The model under review builds one solid part; all positions refer to its coordinate system, in mm. A direction names the side the tool comes from. Coordinates: 2 decimals unless noted, no trailing zeros. Order: outer loops, then holes, each group sorted by start corner. A loop starts at its lowest first (then second) coordinate and runs counter-clockwise, first axis right, second up.
```python
from build123d import *

# Parameters (mm, degrees)
SKETCH_1_W          = 10
SKETCH_1_H          = 10
SKETCH_1_W_2        = 8
SKETCH_1_H_2        = 8
EXTRUDE_1_DEPTH     = 52.5
SKETCH_2_R          = 1.6
CUT_EXTRUDE_1_DEPTH = 54.677276384
SKETCH_3_R          = 1.6
CUT_EXTRUDE_2_DEPTH = 54.677276384
SKETCH_4_R          = 1.6
CUT_EXTRUDE_3_DEPTH = 54.677276384


with BuildPart() as part:
    # ｽｹｯﾁ1 → 押し出し-薄板1 (new body)
    with BuildSketch(Plane.XY):
        Rectangle(SKETCH_1_W, SKETCH_1_H)
        Rectangle(SKETCH_1_W_2, SKETCH_1_H_2, mode=Mode.SUBTRACT)
    extrude(amount=EXTRUDE_1_DEPTH)

    # ｽｹｯﾁ2 → ｶｯﾄ - 押し出し1 (cut, through all)
    with BuildSketch(Plane(origin=(0, 5, 0), x_dir=(1, 0, 0), z_dir=(0, 1, 0))):
        with Locations(Location((0, -5, 0), (0, 0, 180))):
            Circle(SKETCH_2_R)
        with Locations(Location((0, -25, 0), (0, 0, 180))):
            Circle(SKETCH_2_R)
    extrude(amount=-CUT_EXTRUDE_1_DEPTH, mode=Mode.SUBTRACT)

    # ｽｹｯﾁ3 → ｶｯﾄ - 押し出し2 (cut, through all)
    with BuildSketch(Plane(origin=(5, 0, 0), x_dir=(0, 0, -1), z_dir=(1, 0, 0))):
        with Locations(Location((-47.5, 0, 0), (0, 0, 90))):
            Circle(SKETCH_3_R)
        with Locations(Location((-27.5, 0, 0), (0, 0, 90))):
            Circle(SKETCH_3_R)
    extrude(amount=-CUT_EXTRUDE_2_DEPTH, mode=Mode.SUBTRACT)

    # ｽｹｯﾁ4 → ｶｯﾄ - 押し出し3 (cut, through all)
    with BuildSketch(Plane.ZY.offset(5)):
        with Locations(Location((15, 0, 0), (0, 0, 270))):
            Circle(SKETCH_4_R)
    extrude(amount=-CUT_EXTRUDE_3_DEPTH, mode=Mode.SUBTRACT)


solid = part.part
```
(1) For pin 1 Ø1.5 at (x, y) = (0, 3) entering from +Z; pin 2 Ø4 at (y, z) = (0, 27.5) entering from +X, all flat-tipped, find the tip position at first contact; note any pin that passes through.
A:
pin 1: passes through
pin 2: stops at x = 5
(2) Machinability: for faces 1 (the face through (2, -5, 26)), 2 (the face through (-2, 4, 26)), which of the approach directions +Z, -Z, +X, -X, +Y, -Y give a long, thin tool a straight path to every point of the face, cutting with its end or side? Answer none if there is none.
A:
face 1: +Z, -Z, +X, -X, -Y
face 2: +Z, -Z
(3) We need section A-A, the plane z = 5. Write out the cut boundary in (x, y).
A:
outline: (-5, -5) - (-1.6, -5) - (-1.6, -4) - (-4, -4) - (-4, 4) - (-1.6, 4) - (-1.6, 5) - (-5, 5) - close; (1.6, -5) - (5, -5) - (5, 5) - (1.6, 5) - (1.6, 4) - (4, 4) - (4, -4) - (1.6, -4) - close
(4) We need section D-D, the plane x = 0. Write out the cut boundary in (y, z).
A:
outline: (-5, 0) - (-4, 0) - (-4, 3.4) - (-5, 3.4) - close; (-5, 6.6) - (-4, 6.6) - (-4, 23.4) - (-5, 23.4) - close; (-5, 26.6) - (-4, 26.6) - (-4, 52.5) - (-5, 52.5) - close; (4, 0) - (5, 0) - (5, 3.4) - (4, 3.4) - close; (4, 6.6) - (5, 6.6) - (5, 23.4) - (4, 23.4) - close; (4, 26.6) - (5, 26.6) - (5, 52.5) - (4, 52.5) - close
(5) Wall thickness on probe 1 along Z at (x, y) = (-4.65, 0); probe 2 along Z at (x, y) = (0, 4.55); probe 3 along X at (y, z) = (-2.5, 4): over which ranges is each line inside the solid? List them lowest first.
A:
probe 1: z = 0 to 13.4, 16.6 to 25.9, 29.1 to 45.9, 49.1 to 52.5
probe 2: z = 0 to 3.4, 6.6 to 23.4, 26.6 to 52.5
probe 3: x = -5 to -4, 4 to 5
(6) Draft analysis for pull direction X (two halves, no side actions). For faces 3 (the face through (-5, 1, 26)), 4 (the face through (-4.507, 0.208, 16.586)), 5 (the face through (-4, -1, 26)), state which applies: released by +X, released by -X, zero draft, split by the parting line, or undercut.
A:
face 3: released by -X
face 4: zero draft
face 5: undercut
(7) We need section B-B, the plane x = 3.25. Write out the cut boundary in (y, z).
A:
outline: (-5, 0) - (-4, 0) - (-4, 52.5) - (-5, 52.5) - close; (4, 0) - (5, 0) - (5, 52.5) - (4, 52.5) - close
